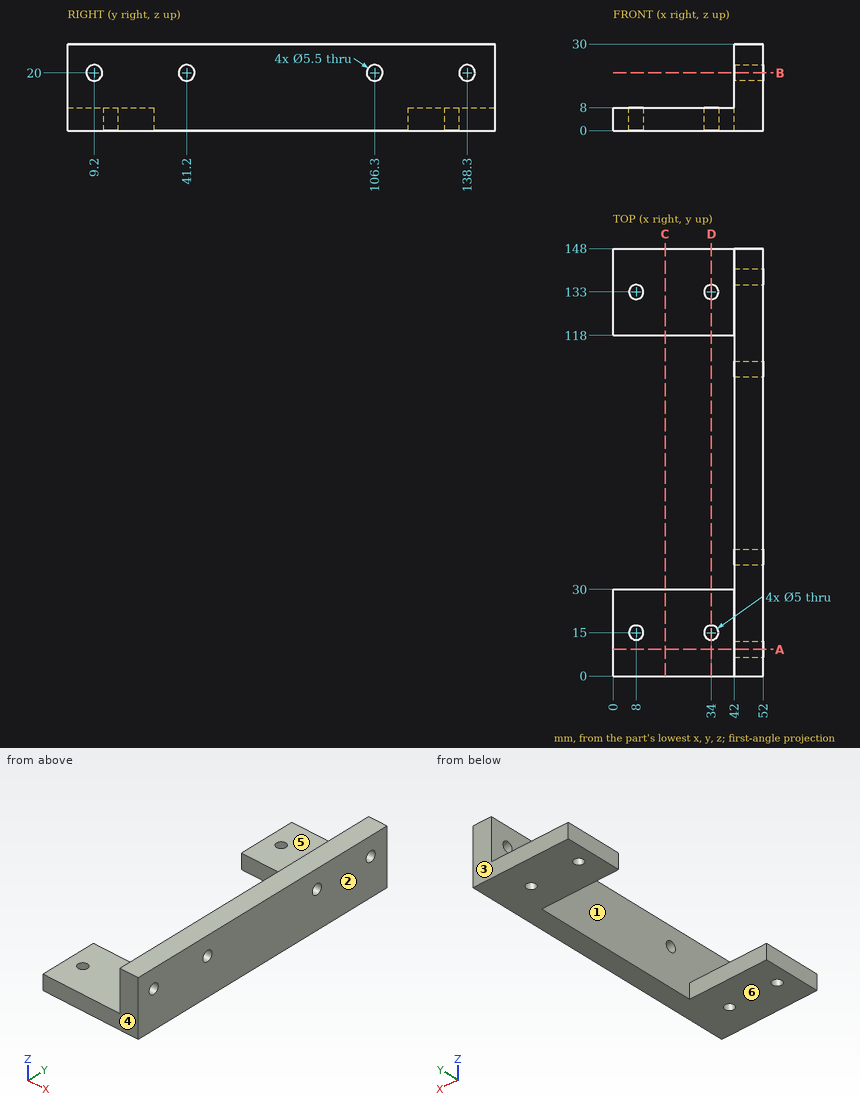
Could you check a few things on this drawing? It's one solid part, dimensions in mm from its lowest x, y, z. A direction names the side the tool comes from. Give positions to 0.01 mm unless a question says otherwise; leave off trailing zeros. Loops run counter-clockwise (first coordinate to the right, second up) from the corner with the lowest first, then second, coordinate; pieces in that order, holes last. Notation, with made-up numbers: (66, 16.5) -> (89, 16.5) arc R15 cw to (89, 40.5) -> close; hole circle Ø8 at (39.5, 52). An arc over 180 degrees is marked (long way). Use one line per item in the form item = value. Start each with the question number.
1) Imagine slicing it at C-C (x = 18). Please give me the cut outline in (y, z).
2) Please list where these lines run through material, in increasing order: line 1 along Y through (x, z) = (46.75, 20); line 2 along Y through (x, z) = (34, 4.5); line 3 along X through (y, z) = (133, 4).
3) For P1, Ø5, axis at y = 9.2, z = 20, coming from the -X side; P2, Ø12, axis at y = 56.5, z = 4, coming from the -X side; P3, Ø6, axis at x = 8, y = 133, coming from the +Z side, each with a flat end and sliding along its axis, tell me the tip position at first contact or that it passes through.
4) Which directions (+Z, -Z, +X, -X, +Y, -Y) give clear straight access to the entire face, cutting with the end or side of a thin tool? Please do the marked faces 5 and 6.
5) Imagine slicing it at B-B (z = 20). Please give me the cut outline in (x, y).
6) Thinking about a two-plate mould opening in Y: for the marked faces 1, 2, 3 and 4, which applies, +Y half, -Y half, draft (parallel to the pull), parting line (faces both ways), or undercut?
7) Imagine slicing it at D-D (x = 34). Please give me the cut outline in (y, z).
8) Imagine slicing it at A-A (y = 9.2). Please give me the cut outline in (x, z), then the cut area to 3 significant figures.
Check values:
q1.outline = (0, 0) -> (30, 0) -> (30, 8) -> (0, 8) -> close; (118, 0) -> (148, 0) -> (148, 8) -> (118, 8) -> close
q2.line_1 = 0 to 6.45, 11.95 to 38.45, 43.95 to 103.55, 109.05 to 135.55, 141.05 to 148
q2.line_2 = 0 to 12.5, 17.5 to 30, 118 to 130.5, 135.5 to 148
q2.line_3 = 0 to 5.5, 10.5 to 31.5, 36.5 to 52
q3.P1 = through
q3.P2 = 42
q3.P3 = 8
q4.face_5 = +Z, -X, +Y, -Y
q4.face_6 = -Z, +X, -X, +Y, -Y
q5.outline = (42, 0) -> (52, 0) -> (52, 6.45) -> (42, 6.45) -> close; (42, 11.95) -> (52, 11.95) -> (52, 38.45) -> (42, 38.45) -> close; (42, 43.95) -> (52, 43.95) -> (52, 103.55) -> (42, 103.55) -> close; (42, 109.05) -> (52, 109.05) -> (52, 135.55) -> (42, 135.55) -> close; (42, 141.05) -> (52, 141.05) -> (52, 148) -> (42, 148) -> close
q6.face_1 = undercut
q6.face_2 = draft
q6.face_3 = +Y half
q6.face_4 = -Y half
q7.outline = (0, 0) -> (12.5, 0) -> (12.5, 8) -> (0, 8) -> close; (17.5, 0) -> (30, 0) -> (30, 8) -> (17.5, 8) -> close; (118, 0) -> (130.5, 0) -> (130.5, 8) -> (118, 8) -> close; (135.5, 0) -> (148, 0) -> (148, 8) -> (135.5, 8) -> close
q8.outline = (0, 0) -> (52, 0) -> (52, 17.25) -> (42, 17.25) -> (42, 8) -> (0, 8) -> close; (42, 22.75) -> (52, 22.75) -> (52, 30) -> (42, 30) -> close
q8.area = 581 mm^2
